from build123d import *

# Parameters (mm, degrees)
SKETCH1_W           = 20
SKETCH1_H           = 12
BOSS_EXTRUDE1_DEPTH = 26
SKETCH2_W           = 10
SKETCH2_H           = 12
BOSS_EXTRUDE2_DEPTH = 8
SKETCH3_R           = 1.6
SKETCH3_R_2         = 1.45
CUT_EXTRUDE1_DEPTH  = 41.049968789
SKETCH4_R           = 1.6
CUT_EXTRUDE2_DEPTH  = 41.049968789
FILLET1_R           = 3
FILLET2_R           = 1
FILLET3_R           = 3
SKETCH5_W           = 9.976745634
SKETCH5_H           = 0.5
SKETCH5_W_2         = 12.25993895
CUT_EXTRUDE3_DEPTH  = 41.049968789
SKETCH6_W           = 5.5
SKETCH6_H           = 30.488056323
CUT_EXTRUDE4_DEPTH  = 0.8
SKETCH7_R           = 1.45
CUT_EXTRUDE5_DEPTH  = 8


with BuildPart() as part:
    # Sketch1 → Boss-Extrude1 (new body)
    with BuildSketch(Plane.XY):
        with Locations((10, -6)):
            Rectangle(SKETCH1_W, SKETCH1_H)
    extrude(amount=BOSS_EXTRUDE1_DEPTH)

    # Sketch2 → Boss-Extrude2 (add)
    with BuildSketch(Plane(origin=(20, 0, 0), x_dir=(0, 0, -1), z_dir=(1, 0, 0))):
        with Locations((-21, -6)):
            Rectangle(SKETCH2_W, SKETCH2_H)
    extrude(amount=BOSS_EXTRUDE2_DEPTH)

    # Sketch3 → Cut-Extrude1 (cut, through all)
    with BuildSketch(Plane.ZY):
        with Locations(Location((5, -6, 0), (0, 0, 270))):
            Circle(SKETCH3_R)
        with Locations(Location((21, -6, 0), (0, 0, 270))):
            Circle(SKETCH3_R_2)
    extrude(amount=-CUT_EXTRUDE1_DEPTH, mode=Mode.SUBTRACT)

    # Sketch4 → Cut-Extrude2 (cut, through all)
    with BuildSketch(Plane(origin=(0, 0, 0), x_dir=(1, 0, 0), z_dir=(0, 1, 0))):
        with Locations(Location((13, -15.5, 0), (0, 0, 270))):
            Circle(SKETCH4_R)
        with Locations(Location((6, -15.5, 0), (0, 0, 270))):
            Circle(SKETCH4_R)
    extrude(amount=-CUT_EXTRUDE2_DEPTH, mode=Mode.SUBTRACT)

    # Fillet1
    fillet1_edges = [part.edges().sort_by_distance(p)[0] for p in [
        (20, -6, 16),
    ]]
    fillet(fillet1_edges, radius=FILLET1_R)

    # Fillet2
    fillet2_edges = [part.edges().sort_by_distance(p)[0] for p in [
        (28, -6, 26),
        (28, -12, 21),
        (28, -6, 16),
        (28, 0, 21),
    ]]
    fillet(fillet2_edges, radius=FILLET2_R)

    # Fillet3
    fillet3_edges = [part.edges().sort_by_distance(p)[0] for p in [
        (10, 0, 0),
        (10, -12, 0),
    ]]
    fillet(fillet3_edges, radius=FILLET3_R)

    # Sketch5 → Cut-Extrude3 (cut, through all)
    with BuildSketch(Plane.ZY):
        with Locations((0.011627183, -11.75)):
            Rectangle(SKETCH5_W, SKETCH5_H)
        with Locations((-1.129969475, -0.25)):
            Rectangle(SKETCH5_W_2, SKETCH5_H)
    extrude(amount=-CUT_EXTRUDE3_DEPTH, mode=Mode.SUBTRACT)

    # Sketch6 → Cut-Extrude4 (cut)
    with BuildSketch(Plane(origin=(0, 0, 0), x_dir=(-1, 0, 0), z_dir=(0, 0, -1))):
        with Locations((-10, -7.868232937)):
            Rectangle(SKETCH6_W, SKETCH6_H)
    extrude(amount=-CUT_EXTRUDE4_DEPTH, mode=Mode.SUBTRACT)

    # Sketch7 → Cut-Extrude5 (cut)
    with BuildSketch(Plane.XY.offset(26)):
        with Locations((10, -6)):
            Circle(SKETCH7_R)
    extrude(amount=-CUT_EXTRUDE5_DEPTH, mode=Mode.SUBTRACT)


solid = part.part
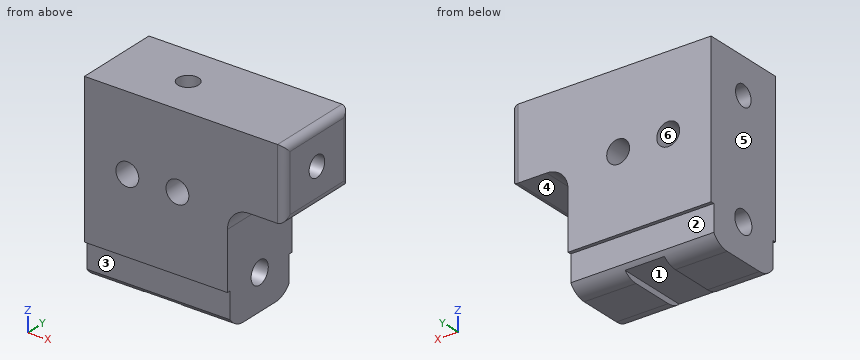
Geometry: final body of the model. Coordinates: model frame, mm. Face numbers are marked on the shaded views. A direction names the side the tool comes from. Give positions to 0.01 mm unless a question says otherwise; leave off trailing zeros. Order: outer loops, then holes, each group sorted by start corner. A loop starts at its lowest first (then second) coordinate and runs counter-clockwise, first axis right, second up. Notation, with made-up numbers: (53, 39) -> (85, 39) arc R12 ccw to (85, 57) -> close; hole circle Ø8 at (-36.75, 89.25). An arc over 180 degrees is marked (long way). Put each result on its own line as item: value.
Q1. Material intervals for L1, parallel to X at y = -8.5, z = 15.25; L2, parallel to X at y = -3.25, z = 15.5; L3, parallel to Z at x = 15.25, y = -6, sorted ascending.
Here are the results:
L1: x = 0 to 4.42, 7.58 to 11.42, 14.58 to 21.02
L2: x = 0 to 4.4, 7.6 to 11.4, 14.6 to 21.34
L3: z = 0 to 3.4, 6.6 to 19.55, 22.45 to 26
Q2. Section C-C, the plane z = 15.5. Return loops of the section in (x, y).
Here are the results:
outline: (0, -12) -> (4.4, -12) -> (4.4, 0) -> (0, 0) -> close; (7.6, -12) -> (11.4, -12) -> (11.4, 0) -> (7.6, 0) -> close; (14.6, -12) -> (21.34, -12) -> (21.34, 0) -> (14.6, 0) -> close
Q3. Section A-A, the plane x = 6. Return loops of the section in (y, z), then the cut area to 3 significant figures.
Here are the results:
outline: (-12, 5) -> (-11.5, 5) -> (-11.5, 1.34) arc R3 ccw to (-9, 0) -> (-3, 0) arc R3 ccw to (-0.5, 1.34) -> (-0.5, 5) -> (0, 5) -> (0, 13.9) -> (-12, 13.9) -> close; (-12, 17.1) -> (0, 17.1) -> (0, 26) -> (-12, 26) -> close; hole circle Ø3.2 at (-6, 5); hole circle Ø2.9 at (-6, 21)
area: 252 mm^2
Q4. Pin query (flat end, axial travel): pin 1 (1.6 mm diameter, centred on x = 8.5, y = -6, fed in from -Z); pin 2 (0.6 mm diameter, centred on x = 6.5, y = -12, fed in from -Z); pin 3 (3 mm diameter, centred on y = -3.5, z = 10, fed in from -X); pin 4 (6 mm diameter, centred on y = -3.5, z = 10.5, fed in from +X). Return the tip coordinate at first contact, or that it passes through.
Here are the results:
pin 1: stops at z = 0.8
pin 2: stops at z = 5
pin 3: stops at x = 0
pin 4: stops at x = 20.04
Q5. Section B-B, the plane y = -3.5. Return loops of the section in (x, z), then the cut area to 3 significant figures.
Here are the results:
outline: (0, 0) -> (7.25, 0) -> (7.25, 0.8) -> (12.75, 0.8) -> (12.75, 0) -> (20, 0) -> (20, 13) arc R3 cw to (23, 16) -> (27, 16) arc R1 ccw to (28, 17) -> (28, 25) arc R1 ccw to (27, 26) -> (0, 26) -> close; hole circle Ø3.2 at (6, 15.5); hole circle Ø3.2 at (13, 15.5)
area: 581 mm^2
Q6. Section D-D, the plane z = 10.75. Return loops of the section in (x, y), then the cut area to 3 significant figures.
Here are the results:
outline: (0, -12) -> (20, -12) -> (20, 0) -> (0, 0) -> close
area: 240 mm^2
Q7. Reachability of the marked faces 1, 2 and 3 from +Z, -Z, +X, -X, +Y, -Y: full face, straight path, thin tool, end or side. Return the list, or none.
Here are the results:
face 1: -Z, +Y, -Y
face 2: -Z, +X, -X, +Y
face 3: -Z, +X, -X, -Y
Q8. Draft query along Z for the marked faces 4, 5 and 6. Return one class per face: released by +Z, released by -Z, zero draft, split by the parting line, or undercut.
Here are the results:
face 4: released by -Z
face 5: zero draft
face 6: undercut
